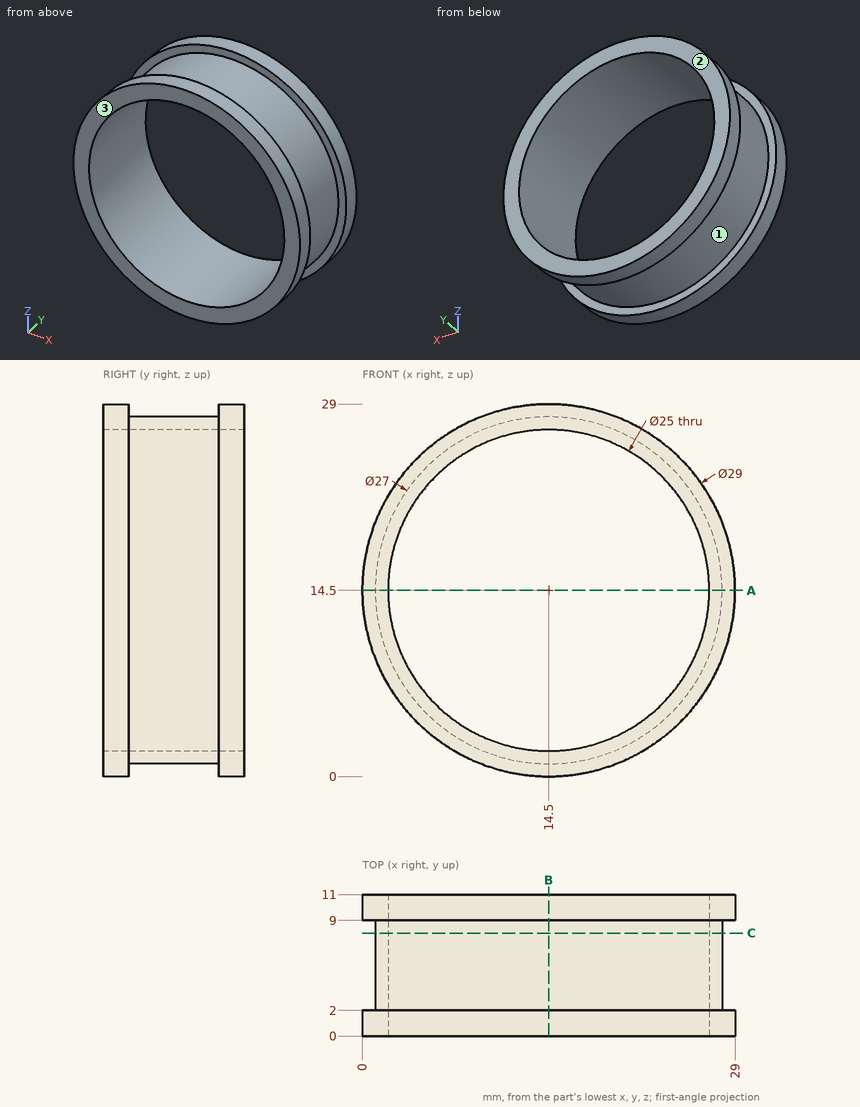
Geometry check sheet. Reference: drawing and pictorial views, mm from the part's lowest x, y, z. Give positions to 0.01 mm unless a question says otherwise; leave off trailing zeros. Write each loop counter-clockwise with the first axis right and the second up, starting at its lowest first coordinate (ties: lowest second). Pieces come first, ordered by that corner, then holes. Notation, with made-up numbers: (59, 18) - (114, 18) arc R8 ccw to (114, 26) - close; hole circle Ø1 at (69.5, 18.25). An arc over 180 degrees is marked (long way). Put each result on its own line as item: value.
Q1. Scan lines: probe 1 along X at (y, z) = (8, 16); probe 2 along Z at (x, y) = (11.5, 8.75); probe 3 along X at (y, z) = (7.75, 14.5). Record each from-to range of solid material in increasing order. Write a range as from..to.
Result:
probe 1: 1.08..2.09, 26.91..27.92
probe 2: 1.34..2.37, 26.63..27.66
probe 3: 1..2, 27..28
Q2. Depth check by flat-ended pin: P1, Ø2, axis at x = 10.5, y = 10, coming from the -Z side; P2, Ø4, axis at y = 5.5, z = 7.5, coming from the -X side. Enter the tip coordinate at first touch or a pass-through.
Result:
P1: z = 0.31
P2: x = 1.96
Q3. Section check C-C on y = 8. Record the cut outline in (x, z), and give its area (3 significant figures).
Result:
outline: circle Ø27 at (14.5, 14.5); hole circle Ø25 at (14.5, 14.5)
area: 81.7 mm2
Q4. Section check B-B on x = 14.5. Record the cut outline in (y, z), and give its area (3 significant figures).
Result:
outline: (0, 0) - (2, 0) - (2, 1) - (9, 1) - (9, 0) - (11, 0) - (11, 2) - (0, 2) - close; (0, 27) - (11, 27) - (11, 29) - (9, 29) - (9, 28) - (2, 28) - (2, 29) - (0, 29) - close
area: 30.0 mm2
Q5. Section check A-A on z = 14.5. Record the cut outline in (x, y), and give its area (3 significant figures).
Result:
outline: (0, 0) - (2, 0) - (2, 11) - (0, 11) - (0, 9) - (1, 9) - (1, 2) - (0, 2) - close; (27, 0) - (29, 0) - (29, 2) - (28, 2) - (28, 9) - (29, 9) - (29, 11) - (27, 11) - close
area: 30.0 mm2
Q6. Mould release check, pull along Y, two halves, no side actions. Record for the marked faces 1, 2 and 3: released by +Y, released by -Y, zero draft, split by the parting line, or undercut.
Result:
face 1: undercut
face 2: released by +Y
face 3: released by -Y
